Could you check a few things on this model? Use its own coordinates, in mm. Face numbers are marked on the shaded views. A direction names the side the tool comes from. Round coordinates to 2 decimals unless told otherwise and drop trailing zeros. Loops run counter-clockwise (first coordinate to the right, second up) from the corner with the lowest first, then second, coordinate; pieces in that order, holes last.
from build123d import *

# Parameters (mm, degrees)
SKETCH2_R           = 15
BOSS_EXTRUDE1_DEPTH = 7.5
SKETCH4_R           = 7.5
BOSS_EXTRUDE2_DEPTH = 10


with BuildPart() as part:
    # Sketch2 → Boss-Extrude1 (new body, symmetric)
    with BuildSketch(Plane(origin=(0, 0, 0), x_dir=(1, 0, 0), z_dir=(0, 1, 0))):
        Circle(SKETCH2_R)
        with BuildLine():
            ThreePointArc((1.936491673, 3.5), (0, -4), (-1.936491673, 3.5))
            Line((-1.936491673, 3.5), (1.936491673, 3.5))
        make_face(mode=Mode.SUBTRACT)
    extrude(amount=BOSS_EXTRUDE1_DEPTH, both=True)

    # Sketch3 → Revolve1 (revolve)
    with BuildSketch(Plane(origin=(0, 0, 0), x_dir=(0, 0, -1), z_dir=(1, 0, 0))):
        with BuildLine():
            ThreePointArc((18.159478483, 6.176007768), (16.745264921, 5.59022133), (16.159478483, 4.176007768))
            Line((16.159478483, 4.176007768), (16.159478483, -4.176007768))
            ThreePointArc((16.159478483, -4.176007768), (16.745264921, -5.59022133), (18.159478483, -6.176007768))
            Line((18.159478483, -6.176007768), (22.413723235, -6.176007768))
            Line((22.413723235, -6.176007768), (22.413723235, -7.5))
            Line((22.413723235, -7.5), (15, -7.5))
            Line((15, -7.5), (15, 7.5))
            Line((15, 7.5), (22.413723235, 7.5))
            Line((22.413723235, 7.5), (22.413723235, 6.176007768))
            Line((22.413723235, 6.176007768), (18.159478483, 6.176007768))
        make_face()
    revolve(axis=Axis((0, 7.5, 0), (0, -1, 0)))

    # Sketch4 → Boss-Extrude2 (add)
    with BuildSketch(Plane(origin=(0, 7.5, 0), x_dir=(1, 0, 0), z_dir=(0, 1, 0))):
        Circle(SKETCH4_R)
        with BuildLine():
            Line((-1.936491673, 3.5), (1.936491673, 3.5))
            ThreePointArc((1.936491673, 3.5), (0, -4), (-1.936491673, 3.5))
        make_face(mode=Mode.SUBTRACT)
    extrude(amount=BOSS_EXTRUDE2_DEPTH)


solid = part.part
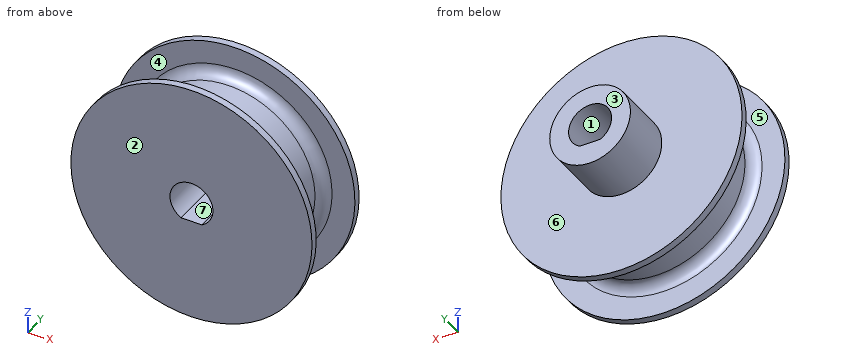
Item 1: If we section it at C-C, the plane y = -0.25: Please give me the cut outline in (x, z).
Results list:
outline: circle Ø32.32 at (0, 0); hole (-1.94, -3.5) - (1.94, -3.5) arc R4 ccw (long way) to start
Item 2: We'd pull the mould along Y, two halves only. Please class the marked faces 1, 2, 3 and 4: released by +Y, released by -Y, zero draft, split by the parting line, or undercut.
Results list:
face 1: zero draft
face 2: released by -Y
face 3: released by +Y
face 4: undercut
Item 3: Will these pins go through, and if not, where does the flat tip stop? pin 1 (22.5 mm diameter, centred on x = 1.5, z = -1, fed in from -Y); pin 2 (12 mm diameter, centred on x = 16.5, z = 3, fed in from +Y); pin 3 (6 mm diameter, centred on y = 4, z = 0.5, fed in from -X); pin 4 (8 mm diameter, centred on x = -7, y = 5.5, fed in from -Z).
Results list:
pin 1: stops at y = -7.5
pin 2: stops at y = 7.5
pin 3: stops at x = -22.41
pin 4: stops at z = -22.2
Item 4: If we section it at D-D, the plane z = 20: Please give me the cut outline in (x, y).
Results list:
outline: (-10.12, -7.5) - (10.12, -7.5) - (10.12, -6.18) - (-10.12, -6.18) - close; (-10.12, 6.18) - (10.12, 6.18) - (10.12, 7.5) - (-10.12, 7.5) - close
Item 5: For the marked faces 5, 6 and 7, which set-ups out of +Z, -Z, +X, -X, +Y, -Y let a thin tool reach every point of the face, with its end or its side?
Results list:
face 5: none
face 6: +Y
face 7: +Y, -Y
Item 6: If we section it at A-A, the plane x = 0: Please give me the cut outline in (y, z), then the cut area to 3 significant figures.
Results list:
outline: (-7.5, -22.41) - (-6.18, -22.41) - (-6.18, -18.16) arc R2 cw to (-4.18, -16.16) - (4.18, -16.16) arc R2 cw to (6.18, -18.16) - (6.18, -22.41) - (7.5, -22.41) - (7.5, -7.5) - (17.5, -7.5) - (17.5, -3.5) - (-7.5, -3.5) - close; (-7.5, 4) - (17.5, 4) - (17.5, 7.5) - (7.5, 7.5) - (7.5, 22.41) - (6.18, 22.41) - (6.18, 18.16) arc R2 cw to (4.18, 16.16) - (-4.18, 16.16) arc R2 cw to (-6.18, 18.16) - (-6.18, 22.41) - (-7.5, 22.41) - close
area: 484 mm2
Item 7: If I drill on line 1 along X through (y, z) = (-1, 0); line 2 along Y through (x, z) = (13.5, 15.5); line 3 along X through (y, z) = (12, 0), over which ranges is the centre line in solid material (lowest first)?
Results list:
line 1: x = -16.16 to -4, 4 to 16.16
line 2: y = -7.5 to -6.18, 6.18 to 7.5
line 3: x = -7.5 to -4, 4 to 7.5
Item 8: If we section it at B-B, the plane z = 0: Please give me the cut outline in (x, y).
Results list:
outline: (-22.41, -7.5) - (-4, -7.5) - (-4, 17.5) - (-7.5, 17.5) - (-7.5, 7.5) - (-22.41, 7.5) - (-22.41, 6.18) - (-18.16, 6.18) arc R2 cw to (-16.16, 4.18) - (-16.16, -4.18) arc R2 cw to (-18.16, -6.18) - (-22.41, -6.18) - close; (4, -7.5) - (22.41, -7.5) - (22.41, -6.18) - (18.16, -6.18) arc R2 cw to (16.16, -4.18) - (16.16, 4.18) arc R2 cw to (18.16, 6.18) - (22.41, 6.18) - (22.41, 7.5) - (7.5, 7.5) - (7.5, 17.5) - (4, 17.5) - close
